Geometry check sheet. Reference: the model listing, model coordinates, mm. Coordinates: 2 decimals unless noted, no trailing zeros. Order: outer loops, then holes, each group sorted by start corner. A loop starts at its lowest first (then second) coordinate and runs counter-clockwise, first axis right, second up. Notation, with made-up numbers: (82.5, 86.5) - (103.5, 86.5) arc R17 cw to (103.5, 112.5) - close; hole circle Ø10 at (-19, 61.25). An arc over 180 degrees is marked (long way). Put each result on its own line as item: value.
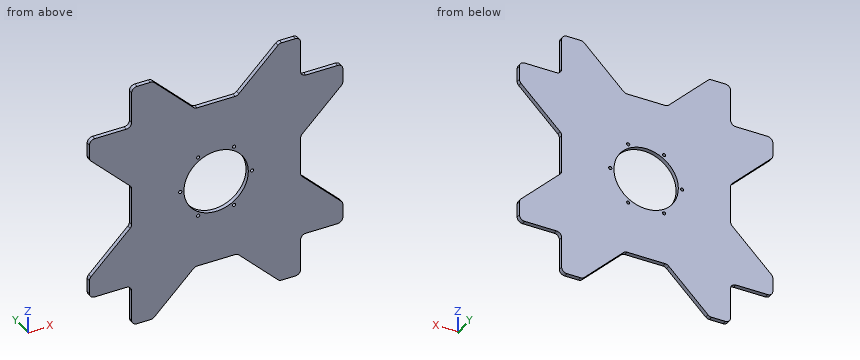
from build123d import *

# Parameters (mm, degrees)
SKETCH_1_W          = 160
SKETCH_1_H          = 160
EXTRUDE_1_DEPTH     = 4
EXTRUDE_2_DEPTH     = 4
FILLET_1_R          = 5
SKETCH_3_R          = 30.5
SKETCH_3_R_2        = 1.5
CUT_EXTRUDE_1_DEPTH = 10


with BuildPart() as part:
    # 草图1 → 凸台-拉伸1 (new body)
    with BuildSketch(Plane(origin=(0, 0, 0), x_dir=(1, 0, 0), z_dir=(0, 1, 0))):
        with Locations((80, 80)):
            Rectangle(SKETCH_1_W, SKETCH_1_H)
    extrude(amount=EXTRUDE_1_DEPTH)

    # 草图2 → 凸台-拉伸2 (add)
    with BuildSketch(Plane(origin=(0, 4, 0), x_dir=(1, 0, 0), z_dir=(0, 1, 0))):
        Polygon((0, 100), (-40, 140), (-40, 160), (0, 160), (0, 200), (20, 200), (60, 160), align=None)
        Polygon((60, 0), (0, 60), (-40, 20), (-40, 0), (0, 0), (0, -40), (20, -40), align=None)
        Polygon((160, 60), (200, 20), (200, 0), (160, 0), (160, -40), (140, -40), (100, 0), align=None)
        Polygon((100, 160), (160, 100), (200, 140), (200, 160), (160, 160), (160, 200), (140, 200), align=None)
    extrude(amount=-EXTRUDE_2_DEPTH)

    # 圆角1
    fillet_1_edges = [part.edges().sort_by_distance(p)[0] for p in [
        (160, 2, -100),
        (200, 2, -140),
        (200, 2, -160),
        (160, 2, -160),
        (160, 2, -200),
        (140, 2, -200),
        (100, 2, -160),
        (140, 2, 40),
        (160, 2, 40),
        (160, 2, 0),
        (200, 2, 0),
        (200, 2, -20),
        (160, 2, -60),
        (100, 2, 0),
        (0, 2, -60),
        (-40, 2, -20),
        (-40, 2, 0),
        (0, 2, 0),
        (0, 2, 40),
        (20, 2, 40),
        (60, 2, 0),
        (20, 2, -200),
        (0, 2, -200),
        (0, 2, -160),
        (-40, 2, -160),
        (-40, 2, -140),
        (0, 2, -100),
        (60, 2, -160),
    ]]
    fillet(fillet_1_edges, radius=FILLET_1_R)

    # 草图3 → 切除-拉伸1 (cut)
    with BuildSketch(Plane(origin=(0, 4, 0), x_dir=(1, 0, 0), z_dir=(0, 1, 0))):
        with Locations(Location((80, 80, 0), (0, 0, 270))):
            Circle(SKETCH_3_R)
        with Locations(Location((97, 109.444863729, 0), (0, 0, 270))):
            Circle(SKETCH_3_R_2)
        with Locations(Location((114, 80, 0), (0, 0, 270))):
            Circle(SKETCH_3_R_2)
        with Locations(Location((97, 50.555136271, 0), (0, 0, 270))):
            Circle(SKETCH_3_R_2)
        with Locations(Location((63, 50.555136271, 0), (0, 0, 270))):
            Circle(SKETCH_3_R_2)
        with Locations(Location((46, 80, 0), (0, 0, 270))):
            Circle(SKETCH_3_R_2)
        with Locations(Location((63, 109.444863729, 0), (0, 0, 270))):
            Circle(SKETCH_3_R_2)
    extrude(amount=-CUT_EXTRUDE_1_DEPTH, mode=Mode.SUBTRACT)


solid = part.part
Q1. Section check C-C on y = 1.6. State how many separate pieces and enclosed holes the cut face has, then the cut area to 3 significant figures.
Answer block:
separate pieces: 1
enclosed holes: 7
area: 35,400 mm^2
Q2. Section check B-B on x = 122. Record the boundary of the cut face in (y, z), then the cut area to 3 significant figures.
Answer block:
outline: (0, -182) - (4, -182) - (4, 22) - (0, 22) - close
area: 816 mm^2
Q3. Section check D-D on x = 31. Record the boundary of the cut face in (y, z).
Answer block:
outline: (0, -189) - (4, -189) - (4, 29) - (0, 29) - close
Q4. Section check A-A on x = 80. Record the boundary of the cut face in (y, z), then the cut area to 3 significant figures.
Answer block:
outline: (0, -160) - (4, -160) - (4, -110.5) - (0, -110.5) - close; (0, -49.5) - (4, -49.5) - (4, 0) - (0, 0) - close
area: 396 mm^2
Q5. Depth check by flat-ended pin: pin 1 Ø2 at (y, z) = (2.5, 20.5) entering from -X; pin 2 Ø1.5 at (x, y) = (20.5, 1.5) entering from +Z; pin 3 Ø1.5 at (x, y) = (4, 2.5) entering from -Z. Enter the tip coordinate at first touch or a pass-through.
Answer block:
pin 1: stops at x = 0
pin 2: stops at z = 39.66
pin 3: stops at z = -199.99
Q6. Thickness scan on L1, parallel to X at y = 3.1, z = -80; L2, parallel to X at y = 0.95, z = -80.5; L3, parallel to X at y = 1.4, z = -173. Record the ranges inside material, lowest first. Write a range as [from, to].
Answer block:
L1: x = [0, 44.5], [47.5, 49.5], [110.5, 112.5], [115.5, 160]
L2: x = [0, 44.59], [47.41, 49.5], [110.5, 112.59], [115.41, 160]
L3: x = [0, 47], [113, 160]
